Here's the drawing with two shaded views (mm, measured from the low corner). I have some questions. A direction names the side the tool comes from. Give positions to 0.01 mm unless a question says otherwise; leave off trailing zeros. Answer as CSV lines item,"result". Start each with the question number.
Q1. Will these pins go through, and if not, where does the flat tip stop? pin 1 Ø3.5 at (y, z) = (1, 4) entering from -X; pin 2 Ø2.5 at (y, z) = (8.5, 3.5) entering from +X; pin 3 Ø5 at (x, y) = (14.425, 9.56) entering from +Z; pin 4 Ø1.5 at (x, z) = (14.5, 2.5) entering from -Y (1 decimal).
Q2. If I drill on line 1 along X through (y, z) = (1.5, 4.25); line 2 along Y through (x, z) = (24.75, 5) (1 decimal); line 3 along Y through (x, z) = (12.5, 4) (1 decimal), over which ranges is the centre line in solid material (lowest first)?
Q3. We'd pull the mould along Y, two halves only. Please class the marked faces 4, 5, 6 and 7: pulls with the +Y half, pulls with the -Y half, needs draft (parallel to the pull), parting line crosses it, or undercut.
Q4. On a 3-axis mill with a long thin cutter (end or side, diameter ignored), from which of +Z, -Z, +X, -X, +Y, -Y can I reach the whole of each face in a straight line? I mean the marked faces 1, 2 and 3. Say none if no direction works.
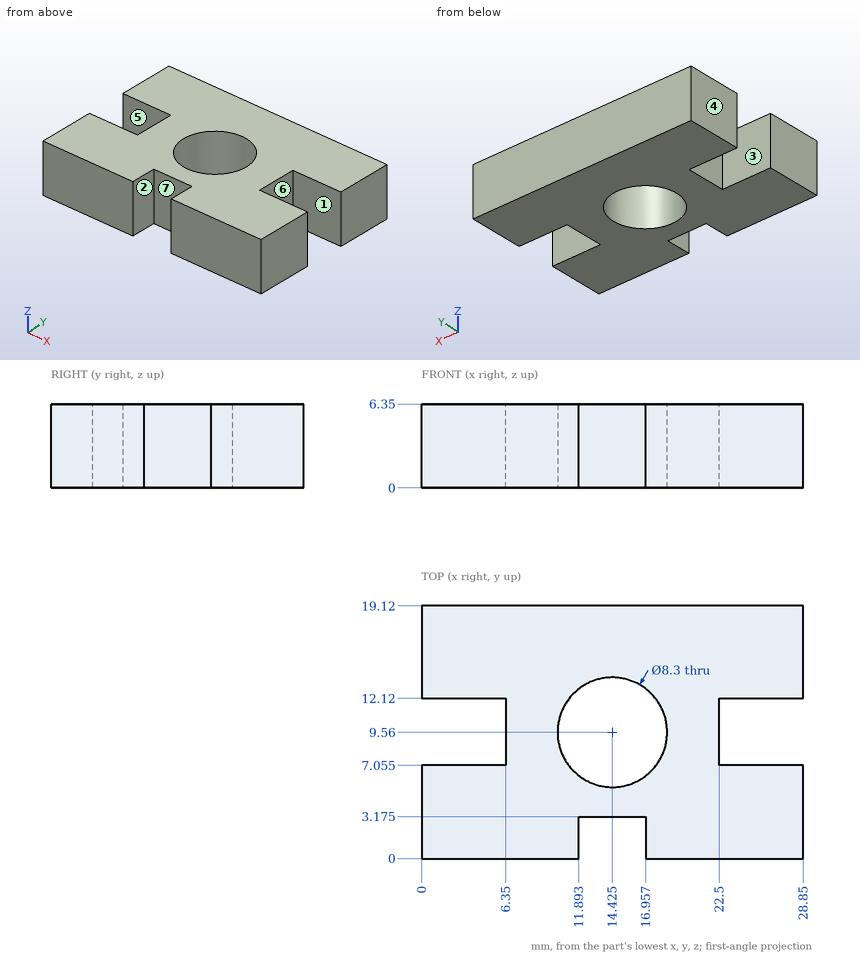
Conclusion:
1,pin 1,"x = 0"
1,pin 2,"x = 22.5"
1,pin 3,"through"
1,pin 4,"y = 3.2"
2,line 1,"0 to 11.89, 16.96 to 28.85"
2,line 2,"0 to 7.1, 12.1 to 19.1"
2,line 3,"3.2 to 5.9, 13.2 to 19.1"
3,face 4,"needs draft"
3,face 5,"undercut"
3,face 6,"undercut"
3,face 7,"pulls with the -Y half"
4,face 1,"+Z, -Z, +X"
4,face 2,"+Z, -Z, -Y"
4,face 3,"+Z, -Z, -X"
